Check sheet for the modelled part. Datum: model origin and axes. Units: mm. A direction names the side the tool comes from. Give positions to 0.01 mm unless a question says otherwise; leave off trailing zeros. Order: outer loops, then holes, each group sorted by start corner. A loop starts at its lowest first (then second) coordinate and runs counter-clockwise, first axis right, second up. Notation, with made-up numbers: M 77,53.25 L 86,53.25 A10 cw 86,60.25 Z; hole C 79.25,51 d11. An arc over 180 degrees is marked long. Return JSON: item names as keys, results as strings. Group by question number.
from build123d import *

# Parameters (mm, degrees)
SKETCH1_R           = 25
BOSS_EXTRUDE1_DEPTH = 65.5
SKETCH2_R           = 15
BOSS_EXTRUDE2_DEPTH = 3
SKETCH3_R           = 6
BOSS_EXTRUDE3_DEPTH = 25
SKETCH4_R           = 19
BOSS_EXTRUDE4_DEPTH = 86.5
SKETCH5_R           = 2.5
CUT_EXTRUDE1_DEPTH  = 10


with BuildPart() as part:
    # Sketch1 → Boss-Extrude1 (new body)
    with BuildSketch(Plane(origin=(0, 0, 0), x_dir=(1, 0, 0), z_dir=(0, 1, 0))):
        Circle(SKETCH1_R)
    extrude(amount=BOSS_EXTRUDE1_DEPTH)

    # Sketch2 → Boss-Extrude2 (add)
    with BuildSketch(Plane(origin=(0, 65.5, 0), x_dir=(1, 0, 0), z_dir=(0, 1, 0))):
        Circle(SKETCH2_R)
    extrude(amount=BOSS_EXTRUDE2_DEPTH)

    # Sketch3 → Boss-Extrude3 (add)
    with BuildSketch(Plane(origin=(0, 68.5, 0), x_dir=(1, 0, 0), z_dir=(0, 1, 0))):
        Circle(SKETCH3_R)
    extrude(amount=BOSS_EXTRUDE3_DEPTH)

    # Sketch4 → Boss-Extrude4 (add)
    with BuildSketch(Plane.XZ):
        Circle(SKETCH4_R)
    extrude(amount=BOSS_EXTRUDE4_DEPTH)

    # Sketch5 → Cut-Extrude1 (cut)
    with BuildSketch(Plane(origin=(0, 65.5, 0), x_dir=(1, 0, 0), z_dir=(0, 1, 0))):
        with Locations((0, 20)):
            Circle(SKETCH5_R)
        with Locations((20, 0)):
            Circle(SKETCH5_R)
        with Locations((0, -20)):
            Circle(SKETCH5_R)
        with Locations((-20, 0)):
            Circle(SKETCH5_R)
    extrude(amount=-CUT_EXTRUDE1_DEPTH, mode=Mode.SUBTRACT)


solid = part.part
1) Sectioned sample at C-C on y = -33. Record the boundary of the cut face in (x, z).
2) Sectioned sample at B-B on z = 0. Record the boundary of the cut face in (x, y), then the cut area to 3 significant figures.
3) Tool access check on faces 4 (the face through (-20, 55.5, 0)), 5 (the face through (0, -86.5, 0)), 6 (the face through (8.767, -42.644, -16.856)). Record the directions out of +Z, -Z, +X, -X, +Y, -Y that give a thin tool (end or side, any length) a straight path to the whole face; none if there is none.
4) Sectioned sample at D-D on z = 11. Record the boundary of the cut face in (x, y).
5) Release check for a two-part mould opening along Z. For faces 1 (the face through (-4, 0, -19)), 2 (the face through (-14.985, 66.979, -0.66)), 3 (the face through (0, 55.5, 20)) record: released by +Z, released by -Z, zero draft, split by the parting line, or undercut.
6) Material ranges on line 1 along X through (y, z) = (59, 0); line 2 along X through (y, z) = (59, 20), recorded low to high.
7) Sectioned sample at A-A on x = 0. Record the boundary of the cut face in (y, z), then the cut area to 3 significant figures.
8) Depth check by flat-ended pin: P1, Ø12, axis at y = -23, z = 19.5, coming from the -X side; P2, Ø5, axis at y = -17.5, z = -6.5, coming from the -X side; P3, Ø8, axis at x = 20, z = 0, coming from the +Y side. Enter the tip coordinate at first touch or a pass-through.
Reply:
{
 "1": {"outline": "C 0,0 d38"},
 "2": {"outline": "M -25,0 L -19,0 L -19,-86.5 L 19,-86.5 L 19,0 L 25,0 L 25,65.5 L 22.5,65.5 L 22.5,55.5 L 17.5,55.5 L 17.5,65.5 L 15,65.5 L 15,68.5 L 6,68.5 L 6,93.5 L -6,93.5 L -6,68.5 L -15,68.5 L -15,65.5 L -17.5,65.5 L -17.5,55.5 L -22.5,55.5 L -22.5,65.5 L -25,65.5 Z", "area": "6,850 mm^2"},
 "3": {"face 4": "+Y", "face 5": "+Z, -Z, +X, -X, -Y", "face 6": "-Y"},
 "4": {"outline": "M -22.45,0 L -15.49,0 L -15.49,-86.5 L 15.49,-86.5 L 15.49,0 L 22.45,0 L 22.45,65.5 L 10.2,65.5 L 10.2,68.5 L -10.2,68.5 L -10.2,65.5 L -22.45,65.5 Z"},
 "5": {"face 1": "zero draft", "face 2": "split by the parting line", "face 3": "undercut"},
 "6": {"line 1": "-25 to -22.5, -17.5 to 17.5, 22.5 to 25", "line 2": "-15 to -2.5, 2.5 to 15"},
 "7": {"outline": "M -86.5,-19 L 0,-19 L 0,-25 L 65.5,-25 L 65.5,-22.5 L 55.5,-22.5 L 55.5,-17.5 L 65.5,-17.5 L 65.5,-15 L 68.5,-15 L 68.5,-6 L 93.5,-6 L 93.5,6 L 68.5,6 L 68.5,15 L 65.5,15 L 65.5,17.5 L 55.5,17.5 L 55.5,22.5 L 65.5,22.5 L 65.5,25 L 0,25 L 0,19 L -86.5,19 Z", "area": "6,850 mm^2"},
 "8": {"P1": "x = -13.37", "P2": "x = -18.57", "P3": "y = 65.5"}
}
